The listing builds one solid part. Answer for the finished solid, in the listing's coordinates (mm). A direction names the side the tool comes from. Coordinates: 2 decimals unless noted, no trailing zeros. Order: outer loops, then holes, each group sorted by start corner. A loop starts at its lowest first (then second) coordinate and runs counter-clockwise, first axis right, second up.
from build123d import *

# Parameters (mm, degrees)
F0_W     = 250
F0_H     = 200
F0_R     = 3.56
F0_R_2   = 2.5
F1_DEPTH = 12.7
F2_R     = 9
F2_R_2   = 5
F3_DEPTH = 6


# Not quite as in the source:
# - a length typed as a fraction of an inch, garbled in the dataset ("3 / 203.2 mm" for 3/8 in), is restored


with BuildPart() as f1:
    # F0 (on Top) → F1 (new body)
    with BuildSketch(Plane.XY):
        Rectangle(F0_W, F0_H)
        with Locations((-44.875, -75)):
            Circle(F0_R, mode=Mode.SUBTRACT)
        with Locations((44.875, -75)):
            Circle(F0_R_2, mode=Mode.SUBTRACT)
        with Locations((11, -11)):
            Circle(F0_R_2, mode=Mode.SUBTRACT)
        with Locations((-11, 11)):
            Circle(F0_R_2, mode=Mode.SUBTRACT)
        with Locations((-44.875, 75)):
            Circle(F0_R, mode=Mode.SUBTRACT)
        with Locations((44.875, 75)):
            Circle(F0_R_2, mode=Mode.SUBTRACT)
    extrude(amount=F1_DEPTH)

    # F2 (on face) → F3 (cut)
    with BuildSketch(Plane.XY.offset(12.7)):
        with Locations((-44.875, 75)):
            Circle(F2_R)
        with Locations((44.875, 75)):
            Circle(F2_R)
        with Locations((-44.875, -75)):
            Circle(F2_R)
        with Locations((44.875, -75)):
            Circle(F2_R)
        with Locations((-11, 11)):
            Circle(F2_R_2)
        with Locations((11, -11)):
            Circle(F2_R_2)
    extrude(amount=-F3_DEPTH, mode=Mode.SUBTRACT)


solid = f1.part
(1) A tool of negligible diameter and unlimited length cuts with its end or side. For faces 1 (the cylindrical face through (-43.232, -78.158, 3.303)), 2 (the cylindrical face through (42.924, 66.214, 9.742)), from which of +Z, -Z, +X, -X, +Y, -Y can it reach the whole face along a straight path? Write none if from no direction.
(2) The mould has two halves that part along X. Classify faces 3 (the flat face through (-41, -75, 6.7)), 4 (the flat face through (125, -1, 6)), 5 (the flat face through (-2, 1, 12.7)): pulls with the +X half, pulls with the -X half, needs draft (parallel to the pull), parting line crosses it, or undercut.
(3) Find section A-A on z = 8.75. Determine the outline of the cut face in (x, y) (3 decimals), then the cut area to 3 significant figures.
(4) Find the intervals of material crossed by probe 1 along Y at (x, z) = (-11, 8.65); probe 2 along X at (y, z) = (75, 4.5) (3 decimals); probe 3 along Y at (x, z) = (11, 5.25), in increasing order.
(5) Given pin 1 Ø6.5 at (x, y) = (44.875, 75) entering from +Z, flat-ended and moving along its own axis, determine where the tip first touches the part or whether it passes through.
Resolved:
1. face 1: +Z, -Z
1. face 2: +Z
2. face 3: undercut
2. face 4: pulls with the +X half
2. face 5: needs draft
3. outline: (-125, -100) - (125, -100) - (125, 100) - (-125, 100) - close; hole circle Ø18 at (-44.875, -75); hole circle Ø18 at (-44.875, 75); hole circle Ø10 at (-11, 11); hole circle Ø10 at (11, -11); hole circle Ø18 at (44.875, -75); hole circle Ø18 at (44.875, 75)
3. area: 48,800 mm2
4. probe 1: y = -100 to 6, 16 to 100
4. probe 2: x = -125 to -48.435, -41.315 to 42.375, 47.375 to 125
4. probe 3: y = -100 to -13.5, -8.5 to 100
5. pin 1: stops at z = 6.7
